The listing builds one solid part. Answer for the finished solid, in the listing's coordinates (mm). A direction names the side the tool comes from. Round coordinates to 2 decimals unless told otherwise and drop trailing zeros. Order: outer loops, then holes, each group sorted by start corner. A loop starts at its lowest first (then second) coordinate and runs counter-clockwise, first axis right, second up. Notation, with made-up numbers: (74.5, 10.5) -> (107.5, 10.5) arc R24 ccw to (107.5, 33.5) -> close; hole circle Ø10 at (31, 12). An arc over 180 degrees is marked (long way). Return JSON: item names as keys, results as strings. Group by question number.
(1) The part is cut by section D-D (y = -1). Determine the outline of the cut face in (x, z).
(2) The part is cut by section B-B (z = 10.75). Determine the outline of the cut face in (x, y).
(3) Determine the mould class of faces 1 (the face through (-13.63, 19.89, 5.16)), 2 (the face through (0, 20.678, 5)), 3 (the face through (-11.97, -3, 9)), 4 (the face through (13.335, 17.358, 3.643)) for opening direction Y: +Y half, -Y half, draft (parallel to the pull), parting line (faces both ways), or undercut.
(4) Which of the six approach directions +Z, -Z, +X, -X, +Y, -Y give full straight-line access (tool end or side, diameter ignored) to faces 5 (the face through (10.631, 13.608, 3.657)), 6 (the face through (13.49, 14.97, 5.16)), 7 (the face through (10.23, -3, 9)), 8 (the face through (0, -3, 13.65))?
(5) Each of these flat-tipped pins is pushed along its axis until it touches: pin 1 (3 mm diameter, centred on x = -0.5, y = 1.5, fed in from +Z); pin 2 (5.5 mm diameter, centred on y = -2, z = 11, fed in from -X); pin 3 (2 mm diameter, centred on y = 17, z = 5, fed in from -X); pin 4 (2.5 mm diameter, centred on y = -3, z = 9, fed in from +X). Where does it stop, or does it pass through?
(6) Consider line 1 (Z direction, x = 6.5, y = -1.25); line 2 (X direction, y = -1.25, z = 10); line 3 (Z direction, x = 9, y = 15.75). Determine where each line is inside the solid, lowest interval first. Write a range as [from, to].
(7) The part is cut by section A-A (x = -6). Determine the outline of the cut face in (y, z), plus the area to 3 significant figures.
(8) The part is cut by section C-C (z = 5.5). Determine the outline of the cut face in (x, y).
Autodesk Inventor part; units mm, degrees
ref_plane "Płaszczyzna konstrukcyjna1" through (-7.6204, -2.8576, 3.15) normal (0, 0, 1) x (1, 0, 0)
ref_plane "Płaszczyzna konstrukcyjna2" through (-10.5274, -25.5076, 4.15) normal (0, 0, -1) x (0, 1, 0)
ref_plane "YZ Plane" through (0, 0, 0) normal (1, 0, 0) x (0, 1, 0)
sketch "Szkic1" plane through (0, 0, 0) normal (0, 0, 1) x (1, 0, 0)
  circle A0 centre (-15.0668, 17.4281) radius 1.6
  circle A1 centre (14.9332, 17.4281) radius 1.6
  circle A2 centre (14.9332, 17.4281) radius 3.25
  circle A3 centre (-15.0668, 17.4281) radius 3.25
  line L0 (14.9332, 14.1781) -> (9.4332, 14.1781)
  line L1 (9.4332, 14.1781) -> (9.4332, 20.6781)
  line L2 (9.4332, 20.6781) -> (14.9332, 20.6781)
  line L3 (14.9332, 20.6781) -> (14.9332, 14.1781)
  line L4 (-15.0668, 14.1781) -> (-9.5668, 14.1781)
  line L5 (-9.5668, 14.1781) -> (-9.5668, 20.6781)
  line L6 (-9.5668, 20.6781) -> (-15.0668, 20.6781)
  line L7 (-15.0668, 20.6781) -> (-15.0668, 14.1781)
  point P0 (0, 0)
  dimension "d0" = 6.5
  dimension "d1" = 6.5
  dimension "d2" = 5.5
  dimension "d3" = 5.5
ref_plane "Płaszczyzna konstrukcyjna1" through (-7.6204, -2.8576, 3.15) normal (0, 0, 1) x (1, 0, 0)
extrude "Wyciągnięcie proste1" add sketch "Szkic1" along normal up to surface (3.15 mm away) contours A0 L7 A3 | A0 L7 A3 | L6 L5 L4 A3 | A1 L3 A2 | A1 L3 A2 | A2 L0 L1 L2
ref_plane "Płaszczyzna konstrukcyjna2" through (-10.5274, -25.5076, 4.15) normal (0, 0, -1) x (0, 1, 0)
sketch "Szkic4" plane through (9.4332, 20.6781, 3.15) normal (0, 0, 1) x (1, 0, 0)
  line L0 (0.5964, -6.1857) -> (-19.4036, -6.1857)
  line L1 (-19.4036, -6.1857) -> (-19.4036, -46.1857)
  line L2 (0.5964, -46.1857) -> (-19.4036, -46.1857)
  line L3 (0.5964, -6.1857) -> (0.5964, -46.1857)
  line L4 (-21.4036, -26.1857) -> (2.5964, -26.1857)
  line L5 (2.5964, -26.1857) -> (2.5964, -21.1857)
  line L6 (2.5964, -21.1857) -> (-21.4036, -21.1857)
  line L7 (-21.4036, -21.1857) -> (-21.4036, -26.1857)
  circle A0 centre (-24.5, -3.25) radius 1.6
  line L8 (-19, -6.5) -> (-24.5, -6.5)
  line L9 (-19, 0) -> (-19, -6.5)
  line L10 (-24.5, 0) -> (-19, 0)
  arc A1 (-24.5, 0) -> (-24.5, -6.5) centre (-24.5, -3.25) ccw
  arc A2 (5.5, -6.5) -> (5.5, 0) centre (5.5, -3.25) ccw
  line L11 (0, 0) -> (5.5, 0)
  line L12 (0, -6.5) -> (0, 0)
  line L13 (5.5, -6.5) -> (0, -6.5)
  circle A3 centre (5.5, -3.25) radius 1.6
  line L14 (-19, 0) -> (0, 0)
  point P0 (-9.4332, -20.6781)
  point P1 (-9.4036, -26.1857)
  point P2 (-9.4036, -46.1857)
  point P3 (0.5964, -21.1857)
  point P4 (0.5964, -6.5)
  point P5 (-19.4036, -6.5)
  point P6 (-19.4036, -21.1857)
  dimension "d15" = 5
  dimension "d16" = 15
  dimension "d17" = 2
extrude "Wyciągnięcie proste4" add sketch "Szkic4" along normal blind 1 contours L3 L13 L12 L0 | L0 L12 L11 A2 L13 L3 | L12 L13 L3 L6 L1 L8 L9 L0 | L0 L9 L14 L12 | L9 L8 L1 L0 | L0 L1 L8 A1 L10 L9 | L6 L5 L4 L3 | L3 L4 L1 L6 | L1 L4 L7 L6
sketch "Szkic5" plane through (9.4332, 20.6781, 4.15) normal (0, 0, 1) x (1, 0, 0)
  line L0 (-21.4036, -21.1857) -> (-21.4036, -26.1857)
  line L1 (2.5964, -21.1857) -> (0.5964, -21.1857)
  line L2 (0.5964, -21.1857) -> (0.5964, -6.5)
  line L3 (0.5964, -6.5) -> (5.5, -6.5)
  arc A0 (5.5, -6.5) -> (5.5, 0) centre (5.5, -3.25) ccw
  line L4 (5.5, 0) -> (-24.5, 0)
  arc A1 (-24.5, 0) -> (-24.5, -6.5) centre (-24.5, -3.25) ccw
  line L5 (-24.5, -6.5) -> (-19.4036, -6.5)
  line L6 (-19.4036, -6.5) -> (-19.4036, -21.1857)
  line L7 (-19.4036, -21.1857) -> (-21.4036, -21.1857)
  line L8 (-21.4036, -21.1857) -> (-21.4036, -26.1857)
  line L9 (-21.4036, -26.1857) -> (2.5964, -26.1857)
  line L10 (2.5964, -26.1857) -> (2.5964, -21.1857)
  circle A2 centre (5.5, -3.25) radius 1.6
  circle A3 centre (-24.5, -3.25) radius 1.6
  line L11 (-21.4036, -26.1857) -> (-19.6036, -26.1857)
  line L12 (-19.6036, -26.1857) -> (-19.6036, -21.1857)
  line L13 (-19.6036, -21.1857) -> (-21.4036, -21.1857)
  line L14 (-21.4036, -21.1857) -> (-21.4036, -26.1857)
  line L15 (2.5964, -26.1857) -> (2.5964, -21.1857)
  line L16 (2.5964, -26.1857) -> (0.7964, -26.1857)
  line L17 (0.7964, -26.1857) -> (0.7964, -21.1857)
  line L18 (0.7964, -21.1857) -> (2.5964, -21.1857)
  line L19 (2.5964, -21.1857) -> (2.5964, -26.1857)
  point P0 (-9.4332, -20.6781)
  point P1 (0.7964, -26.1857)
  dimension "d20" = 1.8
  dimension "d21" = 1.8
extrude "Wyciągnięcie proste5" add sketch "Szkic5" along normal blind 9.5 contours L7 L12 L9 L0 | L17 L1 L10 L9
sketch "Szkic6" plane through (9.4332, 20.6781, 13.65) normal (0, 0, 1) x (1, 0, 0)
  line L0 (-19.6036, -21.1857) -> (-21.4036, -21.1857)
  line L1 (-21.4036, -21.1857) -> (-21.4036, -26.1857)
  line L2 (-21.4036, -26.1857) -> (-19.6036, -26.1857)
  line L3 (-19.6036, -26.1857) -> (-19.6036, -21.1857)
  line L4 (0.7964, -26.1857) -> (2.5964, -26.1857)
  line L5 (2.5964, -26.1857) -> (2.5964, -21.1857)
  line L6 (2.5964, -21.1857) -> (0.7964, -21.1857)
  line L7 (0.7964, -21.1857) -> (0.7964, -26.1857)
  line L8 (-21.4036, -21.1857) -> (-21.4036, -26.1857)
  line L9 (-21.4036, -26.1857) -> (2.5964, -26.1857)
  line L10 (2.5964, -26.1857) -> (2.5964, -21.1857)
  line L11 (2.5964, -21.1857) -> (-21.4036, -21.1857)
  line L12 (-21.4036, -21.1857) -> (-21.4036, -26.1857)
  point P0 (-9.4332, -20.6781)
extrude "Wyciągnięcie proste6" add sketch "Szkic6" along normal blind 2
fillet "Zaokrąglenie3" radius 1 4 edges at (12.0296, -3.0076, 15.65) (-11.9704, -3.0076, 15.65) (12.0296, -3.0076, 3.15) (-11.9704, -3.0076, 3.15)
sketch "Szkic7" plane through (9.4332, 20.6781, 4.15) normal (0, 0, 1) x (1, 0, 0)
  line L0 (0.7964, -26.1857) -> (0.7964, -21.1857)
  line L1 (0.7964, -21.1857) -> (0.5964, -21.1857)
  line L2 (0.5964, -21.1857) -> (0.5964, -6.5)
  line L3 (0.5964, -6.5) -> (5.5, -6.5)
  arc A0 (5.5, -6.5) -> (5.5, 0) centre (5.5, -3.25) ccw
  line L4 (5.5, 0) -> (-24.5, 0)
  arc A1 (-24.5, 0) -> (-24.5, -6.5) centre (-24.5, -3.25) ccw
  line L5 (-24.5, -6.5) -> (-19.4036, -6.5)
  line L6 (-19.4036, -6.5) -> (-19.4036, -21.1857)
  line L7 (-19.4036, -21.1857) -> (-19.6036, -21.1857)
  line L8 (-19.6036, -21.1857) -> (-19.6036, -26.1857)
  line L9 (-19.6036, -26.1857) -> (0.7964, -26.1857)
  circle A2 centre (5.5, -3.25) radius 1.6
  circle A3 centre (-24.5, -3.25) radius 1.6
  line L10 (-19.4036, -6.5) -> (0.5964, -6.5)
  line L11 (-19, -6.5) -> (-19, 0)
  point P0 (-9.4332, -20.6781)
extrude "Wyciągnięcie proste7" add sketch "Szkic7" along normal blind 2 contours L10 L11 L4 A0 L3 | L10 L5 A1 L4 L11
sketch "Szkic8" plane through (9.4332, 20.6781, 6.15) normal (0, 0, 1) x (1, 0, 0)
  circle A0 centre (5.5, -3.25) radius 1.6
  circle A1 centre (-24.5, -3.25) radius 1.6
  circle A2 centre (5.5, -3.25) radius 2.85
  circle A3 centre (-24.5, -3.25) radius 2.85
  line L0 (8.35, -4.8954) -> (5.5, -6.5409)
  line L1 (5.5, -6.5409) -> (2.65, -4.8954)
  line L2 (2.65, -4.8954) -> (2.65, -1.6046)
  line L3 (2.65, -1.6046) -> (5.5, 0.0409)
  line L4 (5.5, 0.0409) -> (8.35, -1.6046)
  line L5 (8.35, -1.6046) -> (8.35, -4.8954)
  line L6 (5.5, 0) -> (-24.5, 0)
  arc A4 (-24.5, 0) -> (-24.5, -6.5) centre (-24.5, -3.25) ccw
  line L7 (-24.5, -6.5) -> (5.5, -6.5)
  arc A5 (5.5, -6.5) -> (5.5, 0) centre (5.5, -3.25) ccw
  circle A6 centre (-24.5, -3.25) radius 1.6
  circle A7 centre (5.5, -3.25) radius 1.6
  line L8 (-27.35, -1.6046) -> (-24.5, 0.0409)
  line L9 (-24.5, 0.0409) -> (-21.65, -1.6046)
  line L10 (-21.65, -1.6046) -> (-21.65, -4.8954)
  line L11 (-21.65, -4.8954) -> (-24.5, -6.5409)
  line L12 (-24.5, -6.5409) -> (-27.35, -4.8954)
  line L13 (-27.35, -4.8954) -> (-27.35, -1.6046)
  point P0 (-9.4332, -20.6781)
  point P1 (8.35, -3.25)
  point P2 (-27.35, -3.25)
  point P3 (-24.5722, -0.0008)
  point P4 (-27.2778, -1.5629)
  point P5 (-27.35, -1.688)
  point P6 (-27.35, -4.812)
  point P7 (-27.2778, -4.9371)
  point P8 (-24.5722, -6.4992)
  point P9 (5.5722, -6.4992)
  point P10 (8.2778, -4.9371)
  point P11 (8.35, -4.812)
  point P12 (8.35, -1.688)
  point P13 (8.2778, -1.5629)
  point P14 (5.5722, -0.0008)
  dimension "d29" = 5.7
  dimension "d30" = 5.7
extrude "Wyciągnięcie proste8" cut sketch "Szkic8" against normal blind 2 contours A0 | A1 | A2 | L5 A5 L0 A2 | A2 L4 A5 L5 | L5 A5 | A2 L3 L6 A5 L4 | L4 A5 | L0 A5 L7 L1 A2 | L0 A5 | A5 L4 L5 | L5 L0 A5 | A2 L2 L3 | A5 L6 L3 L4 | L1 L2 A2 | L0 L1 L7 A5 | L9 A3 L8 A4 L6 | L6 A4 L8 L9 | L11 L12 A4 L7 | L7 A4 L12 A3 L11 | L9 L10 A3 | A3 | A3 L10 L11 | L8 A4 | A3 L13 A4 L8 | A4 L12 | L12 A4 L13 A3 | A4 L13 L8 | L13 A4 | L12 L13 A4
sketch "Szkic10" plane through (0, 0, 0) normal (0, 0, -1) x (-1, 0, 0)
  line L0 (9.5668, 14.1781) -> (9.5668, 20.6781)
  line L1 (15.0668, 14.1781) -> (9.5668, 14.1781)
  arc A0 (15.0668, 14.1781) -> (15.0668, 20.6781) centre (15.0668, 17.4281) ccw
  line L2 (9.5668, 20.6781) -> (15.0668, 20.6781)
  circle A1 centre (15.0668, 17.4281) radius 1.6
  line L3 (-14.9332, 20.6781) -> (-9.4332, 20.6781)
  arc A2 (-14.9332, 20.6781) -> (-14.9332, 14.1781) centre (-14.9332, 17.4281) ccw
  line L4 (-9.4332, 14.1781) -> (-14.9332, 14.1781)
  line L5 (-9.4332, 20.6781) -> (-9.4332, 14.1781)
  circle A3 centre (-14.9332, 17.4281) radius 1.6
  point P0 (0, 0)
extrude "Wyciągnięcie proste9" cut sketch "Szkic10" against normal up to surface (3.15 mm away)
fillet "Zaokrąglenie4" radius 2 2 edges at (-9.9704, 14.1781, 3.65) (10.0296, 14.1781, 3.65)
fillet "Zaokrąglenie5" radius 0.2 2 edges at (-9.9704, -0.5076, 3.65) (10.0296, -0.5076, 3.65)
properties part number "trzymacz"
Answer below:
{
 "1": {"outline": "(-11.97, 4.15) arc R1 ccw to (-10.97, 3.15) -> (11.03, 3.15) arc R1 ccw to (12.03, 4.15) -> (12.03, 14.65) arc R1 ccw to (11.03, 15.65) -> (-10.97, 15.65) arc R1 ccw to (-11.97, 14.65) -> close; hole (-10.17, 4.15) -> (10.23, 4.15) -> (10.23, 13.65) -> (-10.17, 13.65) -> close"},
 "2": {"outline": "(-11.97, -5.51) -> (-10.17, -5.51) -> (-10.17, -0.51) -> (-11.97, -0.51) -> close; (10.23, -5.51) -> (12.03, -5.51) -> (12.03, -0.51) -> (10.23, -0.51) -> close"},
 "3": {"face 1": "undercut", "face 2": "+Y half", "face 3": "draft", "face 4": "undercut"},
 "4": {"face 5": "+Z, -Z, +X", "face 6": "+Z, +X", "face 7": "-Y", "face 8": "+Y, -Y"},
 "5": {"pin 1": "stops at z = 4.15", "pin 2": "stops at x = -11.97", "pin 3": "stops at x = -18.32", "pin 4": "stops at x = 12.03"},
 "6": {"line 1": "z = [3.15, 4.15], [13.65, 15.65]", "line 2": "x = [-11.97, -10.17], [10.23, 12.03]", "line 3": "z = [3.15, 6.15]"},
 "7": {"outline": "(-5.51, 3.15) -> (20.68, 3.15) -> (20.68, 6.15) -> (14.18, 6.15) -> (14.18, 4.15) -> (-5.51, 4.15) -> close; (-5.51, 13.65) -> (-0.51, 13.65) -> (-0.51, 15.65) -> (-5.51, 15.65) -> close", "area": "49.2 mm²"},
 "8": {"outline": "(-15, 14.18) -> (14.86, 14.18) -> (12.08, 15.78) -> (12.08, 19.07) -> (14.86, 20.68) -> (-15, 20.68) -> (-12.22, 19.07) -> (-12.22, 15.78) -> close; (-11.97, -5.51) -> (-10.17, -5.51) -> (-10.17, -0.51) -> (-11.97, -0.51) -> close; (10.23, -5.51) -> (12.03, -5.51) -> (12.03, -0.51) -> (10.23, -0.51) -> close"}
}
